from build123d import *

# Parameters (mm, degrees)
SKETCH1_W           = 36.5
SKETCH1_H           = 24
BOSS_EXTRUDE1_DEPTH = 2.5
SKETCH2_W           = 36.5
SKETCH2_H           = 3
BOSS_EXTRUDE2_DEPTH = 23
SKETCH3_R           = 3
SKETCH3_R_2         = 1.55
CUT_EXTRUDE2_DEPTH  = 51.581617214
SKETCH6_R           = 1.5
CUT_EXTRUDE4_DEPTH  = 50.368512232
CUT_EXTRUDE5_REACH  = 52.582


with BuildPart() as part:
    # Sketch1 → Boss-Extrude1 (new body)
    with BuildSketch(Plane(origin=(0, 0, 0), x_dir=(1, 0, 0), z_dir=(0, 1, 0))):
        with Locations((18.25, 12)):
            Rectangle(SKETCH1_W, SKETCH1_H)
    extrude(amount=BOSS_EXTRUDE1_DEPTH)

    # Sketch2 → Boss-Extrude2 (add)
    with BuildSketch(Plane(origin=(0, 2.5, 0), x_dir=(1, 0, 0), z_dir=(0, 1, 0))):
        with Locations((18.25, 1.5)):
            Rectangle(SKETCH2_W, SKETCH2_H)
        with Locations((18.25, 22.5)):
            Rectangle(SKETCH2_W, SKETCH2_H)
    extrude(amount=BOSS_EXTRUDE2_DEPTH)

    # Sketch3 → Cut-Extrude2 (cut, through all)
    with BuildSketch(Plane.XY):
        with Locations((25.5, 13.75)):
            Circle(SKETCH3_R)
        with BuildLine():
            Line((36.5, 2.5), (36.5, 22.497165255))
            Line((36.5, 22.497165255), (24.17707002, 16.442555713))
            ThreePointArc((24.17707002, 16.442555713), (27.086065897, 16.29644752), (28.5, 13.75))
            ThreePointArc((28.5, 13.75), (26.893321833, 11.093187197), (23.794230487, 11.282136477))
            Line((23.794230487, 11.282136477), (36.5, 2.5))
        make_face()
        with Locations((6.9, 22.65)):
            Circle(SKETCH3_R_2)
        with Locations((6.9, 5.05)):
            Circle(SKETCH3_R_2)
    extrude(amount=-CUT_EXTRUDE2_DEPTH, mode=Mode.SUBTRACT)

    # Sketch6 → Cut-Extrude4 (cut, through all)
    with BuildSketch(Plane(origin=(0, 2.5, 0), x_dir=(1, 0, 0), z_dir=(0, 1, 0))):
        with Locations(Location((4, 19, 0), (0, 0, 270))):
            Circle(SKETCH6_R)
        with Locations(Location((32.5, 19, 0), (0, 0, 90))):
            Circle(SKETCH6_R)
        with Locations(Location((32.5, 5, 0), (0, 0, 270))):
            Circle(SKETCH6_R)
        with Locations(Location((4, 5, 0), (0, 0, 90))):
            Circle(SKETCH6_R)
    extrude(amount=-CUT_EXTRUDE4_DEPTH, mode=Mode.SUBTRACT)

    # Sketch8 → Cut-Extrude5 (cut, up to next)
    with BuildSketch(Plane(origin=(0, 0, -24), x_dir=(-1, 0, 0), z_dir=(0, 0, -1)), mode=Mode.PRIVATE) as cut_extrude5_sk1:
        with BuildLine():
            Line((-24.564111876, 10.75), (-14.5, 10.75))
            ThreePointArc((-14.5, 10.75), (-11.5, 13.75), (-14.5, 16.75))
            Line((-14.5, 16.75), (-24.802810523, 16.75))
            Line((-24.802810523, 16.75), (-24.17707002, 16.442555713))
            ThreePointArc((-24.17707002, 16.442555713), (-22.508221795, 13.971953085), (-23.794230487, 11.282136477))
            Line((-23.794230487, 11.282136477), (-24.564111876, 10.75))
        make_face()
    cut_extrude5_tool1 = extrude(cut_extrude5_sk1.sketch, amount=-CUT_EXTRUDE5_REACH, mode=Mode.PRIVATE) & part.part
    add(cut_extrude5_tool1.solids().sort_by_distance((17.630744, 13.752153, -24))[0], mode=Mode.SUBTRACT)


solid = part.part
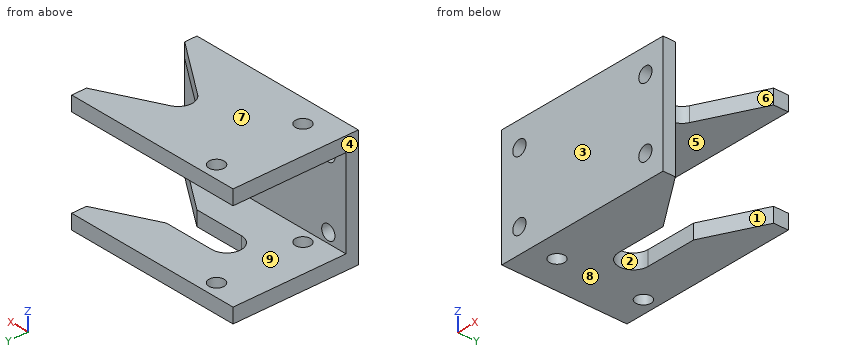
Input: part model. Units: mm. Frame: model coordinates. Face numbers are marked on the shaded views. A direction names the side the tool comes from. Coordinates: 2 decimals unless noted, no trailing zeros. Loops run counter-clockwise (first coordinate to the right, second up) from the corner with the lowest first, then second, coordinate; pieces in that order, holes last. Notation, with made-up numbers: (-21.5, 39) -> (29.5, 39) arc R24 ccw to (29.5, 71) -> close; hole circle Ø8 at (49.25, 33.5). An arc over 180 degrees is marked (long way). Write item = value, one per line. Start each with the question number.
Item 1: Mould query, pull axis Z, two halves, no side actions, for the marked faces 6, 7, 8 and 9. Classes: pulls with the +Z half, pulls with the -Z half, needs draft (parallel to the pull), parting line crosses it, or undercut.
Item 2: First-contact query: P1, Ø2.5, axis at x = 6.9, y = 22.65, coming from the +Z side; P2, Ø1.5, axis at x = 4.5, z = -10, coming from the -Y side. Flat tips, straight axial feed; report the tip coordinate or a pass-through.
Item 3: Cut plane A-A, the plane x = 4. Return loops of the section in (y, z).
Item 4: Material intervals for line 1 (Y direction, x = 6.9, z = -2.15); line 2 (X direction, y = 1.95, z = -5); line 3 (Z direction, x = 27, y = 18), sorted ascending.
Item 5: Reachability of the marked faces 1, 2, 3, 4 and 5 from +Z, -Z, +X, -X, +Y, -Y: full face, straight path, thin tool, end or side. Return the list, or none.
Item 6: Cut plane D-D, the plane z = -2.5. Return loops of the section in (x, y).
Item 7: Cut plane B-B, the plane z = -19. Return loops of the section in (x, y), plus the area to 4 significant figures.
Item 8: Cut plane C-C, the plane y = 13.75. Return loops of the section in (x, z).
Ans:
q1.face_6 = needs draft
q1.face_7 = pulls with the +Z half
q1.face_8 = pulls with the -Z half
q1.face_9 = undercut
q2.P1 = through
q2.P2 = 0
q3.outline = (0, -24) -> (25.5, -24) -> (25.5, -21) -> (2.5, -21) -> (2.5, -20.5) -> (0, -20.5) -> close; (0, -17.5) -> (2.5, -17.5) -> (2.5, -6.5) -> (0, -6.5) -> close; (0, -3.5) -> (2.5, -3.5) -> (2.5, -3) -> (25.5, -3) -> (25.5, 0) -> (0, 0) -> close
q4.line_1 = 0 to 3.5, 6.6 to 21.1, 24.2 to 25.5
q4.line_2 = 0 to 2.5, 5.5 to 31, 34 to 36.5
q4.line_3 = -24 to -21, -3 to 0
q5.face_1 = +Z, -Z, +X
q5.face_2 = -Z, +X
q5.face_3 = +Z, -Z, +X, -X, -Y
q5.face_4 = +Z, -Z, -X, +Y, -Y
q5.face_5 = +X, -X, +Y
q6.outline = (0, 0) -> (36.5, 0) -> (36.5, 2.5) -> (23.79, 11.28) arc R3 cw to (24.18, 16.44) -> (36.5, 22.5) -> (36.5, 25.5) -> (0, 25.5) -> close; hole circle Ø3.1 at (6.9, 5.05); hole circle Ø3.1 at (6.9, 22.65)
q7.outline = (0, 0) -> (2.5, 0) -> (2.5, 2.5) -> (0, 2.5) -> close; (5.5, 0) -> (31, 0) -> (31, 2.5) -> (5.5, 2.5) -> close; (34, 0) -> (36.5, 0) -> (36.5, 2.5) -> (34, 2.5) -> close
q7.area = 76.25 mm²
q8.outline = (0, -24) -> (11.5, -24) -> (11.5, -21) -> (0, -21) -> close; (0, -3) -> (22.5, -3) -> (22.5, 0) -> (0, 0) -> close
